from build123d import *

# Parameters (mm, degrees)
SKETCH_W        = 460
SKETCH_H        = 360
PAD_DEPTH       = 5
SKETCH001_R     = 5
POCKET_DEPTH    = 5.001
SKETCH002_W     = 160
SKETCH002_H     = 30
POCKET001_DEPTH = 5.001


with BuildPart() as part:
    # Sketch → Pad (new body)
    with BuildSketch(Plane.XY):
        with Locations((230, 180)):
            Rectangle(SKETCH_W, SKETCH_H)
    extrude(amount=PAD_DEPTH)

    # Sketch001 (on Face6 of Pad) → Pocket (cut, through all)
    with BuildSketch(Plane.XY.offset(5)):
        with Locations((15, 180)):
            Circle(SKETCH001_R)
    extrude(amount=-POCKET_DEPTH, mode=Mode.SUBTRACT)

    # Sketch002 (on Face5 of Pocket) → Pocket001 (cut, through all)
    with BuildSketch(Plane.XY.offset(5)):
        with Locations((110, 15)):
            Rectangle(SKETCH002_W, SKETCH002_H)
    extrude(amount=-POCKET001_DEPTH, mode=Mode.SUBTRACT)


solid = part.part
Input: part model. Units: mm. Frame: model coordinates. Coordinates: 2 decimals unless noted, no trailing zeros. Order: outer loops, then holes, each group sorted by start corner. A loop starts at its lowest first (then second) coordinate and runs counter-clockwise, first axis right, second up. Notation, with made-up numbers: M 56,-11.75 L 93,-11.75 A20 cw 93,7.25 Z; hole C 41,-32 d1. An arc over 180 degrees is marked long. One line per question, with ' | ' between items.
Item 1: Section A-A (y = 180). Output: boundary loops of the cut face in (x, z).
Geometry results:
outline: M 0,0 L 10,0 L 10,5 L 0,5 Z; M 20,0 L 460,0 L 460,5 L 20,5 Z
Item 2: Section C-C (x = 15). Output: boundary loops of the cut face in (y, z).
Geometry results:
outline: M 0,0 L 175,0 L 175,5 L 0,5 Z; M 185,0 L 360,0 L 360,5 L 185,5 Z
Item 3: Draft query along X for faces 1 (the cylindrical face through (14.349, 184.957, 2.535)), 2 (the flat face through (227, 183, 0)). Return one class per face: released by +X, released by -X, zero draft, split by the parting line, or undercut.
Geometry results:
face 1: undercut | face 2: zero draft
Item 4: Ray query, line 1 along Y through (x, z) = (15, 3.5); line 2 along Y through (x, z) = (156, 1.5). Return the intervals inside material, ascending.
Geometry results:
line 1: y = 0 to 175, 185 to 360 | line 2: y = 30 to 360
Item 5: Section B-B (z = 3.6). Output: boundary loops of the cut face in (x, y).
Geometry results:
outline: M 0,0 L 30,0 L 30,30 L 190,30 L 190,0 L 460,0 L 460,360 L 0,360 Z; hole C 15,180 d10
Item 6: Pin query (flat end, axial travel): pin 1 (2.5 mm diameter, centred on x = 145.5, z = 3.5, fed in from -Y). Return the tip coordinate at first contact, or that it passes through.
Geometry results:
pin 1: stops at y = 30
